Input: part model. Units: mm. Frame: model coordinates. Face numbers are marked on the shaded views. Coordinates: 2 decimals unless noted, no trailing zeros. Loops run counter-clockwise (first coordinate to the right, second up) from the corner with the lowest first, then second, coordinate; pieces in that order, holes last.
(1) Section B-B, the plane z = -1866.5. Return loops of the section in (x, y).
(2) Mould query, pull axis Z, two halves, no side actions, for the marked faces 1, 2 and 3. Classes: released by +Z, released by -Z, zero draft, split by the parting line, or undercut.
(3) Section C-C, the plane y = 150.5. Return loops of the section in (x, z), then the cut area to 3 significant figures.
(4) Contact query for flat-ended pins moving along their axis: P1, Ø6, axis at x = -238.5, z = -1429, coming from the +Y side; P2, Ø9, axis at x = 432.5, z = -2165, coming from the -Y side; P3, Ø1, axis at x = 249.5, z = -976, coming from the -Y side; P4, Ø20, axis at x = -436, y = -102.5, coming from the +Z side. Output: stop coordinate, or through.
(5) Section A-A, the plane y = -201.5. Give the number of separate pieces and of enclosed holes in the cut face, then the cut area to 3 significant figures.
(6) Section D-D, the plane x = -172. Return loops of the section in (y, z), then the cut area to 3 significant figures.
(7) Line query: L1, parallel to Z at x = 66, y = 171.5; L2, parallel to Y at x = 334.5, z = -1180; L3, parallel to Z at x = -41, y = -112.5. Output: solid intervals per line, ascending.
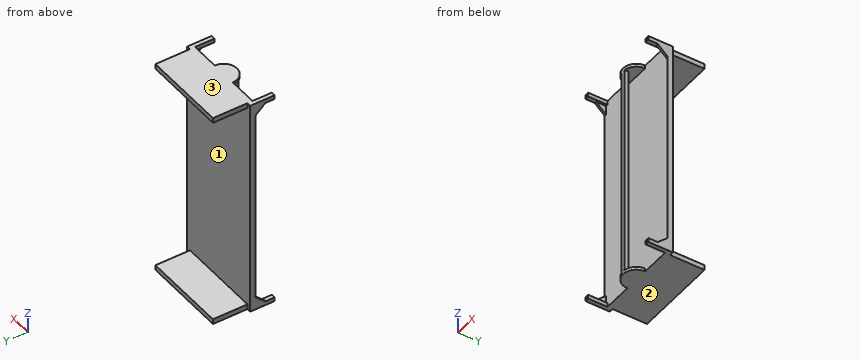
```python
from build123d import *

# Parameters (mm, degrees)
SKETCH1_W                = 40
SKETCH1_H                = 10
BOSS_EXTRUDE1_DEPTH      = 50
BOSS_EXTRUDE2_DEPTH      = 340
BOSS_EXTRUDE2_DEPTH_BACK = 50
SKETCH1_4_W              = 40
SKETCH1_4_H              = 40
BOSS_EXTRUDE3_DEPTH      = 240
BOSS_EXTRUDE4_DEPTH      = 20
BOSS_EXTRUDE5_DEPTH      = 20
SKETCH5_W                = 30
SKETCH5_H                = 30
CUT_EXTRUDE1_DEPTH       = 200
BOSS_EXTRUDE6_DEPTH      = 30
BOSS_EXTRUDE7_START      = -30
BOSS_EXTRUDE7_DEPTH      = 30
BOSS_EXTRUDE8_DEPTH      = 20
BOSS_EXTRUDE8_DEPTH_BACK = 20


with BuildPart() as part:
    # Sketch1 → Boss-Extrude1 (new body)
    with BuildSketch(Plane(origin=(0, 0, 0), x_dir=(1, 0, 0), z_dir=(0, 1, 0))):
        Polygon((-457.5, 50), (-417.5, 50), (417.5, 50), (457.5, 50), (457.5, 2130), (417.5, 2130), (-417.5, 2130), (-457.5, 2130), align=None)
        with Locations((-437.5, 45)):
            Rectangle(SKETCH1_W, SKETCH1_H)
        with Locations((437.5, 45)):
            Rectangle(SKETCH1_W, SKETCH1_H)
        with Locations((437.5, 2135)):
            Rectangle(SKETCH1_W, SKETCH1_H)
        with Locations((-437.5, 2135)):
            Rectangle(SKETCH1_W, SKETCH1_H)
    extrude(amount=-BOSS_EXTRUDE1_DEPTH)

    # Sketch1_3 → Boss-Extrude2 (add, two sides: drawn at the far end of the back side and taken through both)
    with BuildSketch(Plane(origin=(0, 0, 0), x_dir=(1, 0, 0), z_dir=(0, 1, 0)).offset(-BOSS_EXTRUDE2_DEPTH_BACK)):
        Polygon((-417.5, 50), (-417.5, 40), (-417.5, 0), (417.5, 0), (417.5, 40), (417.5, 50), align=None)
        Polygon((-417.5, 2140), (-417.5, 2130), (417.5, 2130), (417.5, 2140), (417.5, 2180), (-417.5, 2180), align=None)
    extrude(amount=BOSS_EXTRUDE2_DEPTH + BOSS_EXTRUDE2_DEPTH_BACK)

    # Sketch1_4 → Boss-Extrude3 (add)
    with BuildSketch(Plane(origin=(0, 0, 0), x_dir=(1, 0, 0), z_dir=(0, 1, 0))):
        with Locations((437.5, 2160)):
            Rectangle(SKETCH1_4_W, SKETCH1_4_H)
        with Locations((-437.5, 2160)):
            Rectangle(SKETCH1_4_W, SKETCH1_4_H)
        with Locations((-437.5, 20)):
            Rectangle(SKETCH1_4_W, SKETCH1_4_H)
        with Locations((437.5, 20)):
            Rectangle(SKETCH1_4_W, SKETCH1_4_H)
    extrude(amount=-BOSS_EXTRUDE3_DEPTH)

    # Sketch3 → Boss-Extrude4 (add)
    with BuildSketch(Plane(origin=(457.5, 0, 0), x_dir=(0, 0, -1), z_dir=(1, 0, 0))):
        Polygon((40, -50), (40, -150), (130, -50), align=None)
        Polygon((2140, -50), (2050, -50), (2140, -150), align=None)
    extrude(amount=-BOSS_EXTRUDE4_DEPTH)

    # Sketch4 → Boss-Extrude5 (add)
    with BuildSketch(Plane(origin=(-457.5, 0, -45.75), x_dir=(0, 0, -1), z_dir=(1, 0, 0))):
        Polygon((2094.25, -50), (2004.25, -50), (2094.25, -150), align=None)
        Polygon((-5.75, -50), (-5.75, -150), (84.25, -50), align=None)
    extrude(amount=BOSS_EXTRUDE5_DEPTH)

    # Sketch5 → Cut-Extrude1 (cut)
    with BuildSketch(Plane.XZ.offset(240)):
        with Locations((-437.5, -2160)):
            Rectangle(SKETCH5_W, SKETCH5_H)
        with Locations((437.5, -2160)):
            Rectangle(SKETCH5_W, SKETCH5_H)
        with Locations((437.5, -20)):
            Rectangle(SKETCH5_W, SKETCH5_H)
        with Locations((-437.5, -20)):
            Rectangle(SKETCH5_W, SKETCH5_H)
    extrude(amount=-CUT_EXTRUDE1_DEPTH, mode=Mode.SUBTRACT)

    # Sketch6 → Boss-Extrude6 (add)
    with BuildSketch(Plane.XY):
        with BuildLine():
            Line((130, -50), (-130, -50))
            ThreePointArc((-130, -50), (0, -180), (130, -50))
        make_face()
    extrude(amount=-BOSS_EXTRUDE6_DEPTH)

    # Sketch7 → Boss-Extrude7 (add)
    with BuildSketch(Plane(origin=(0, 0, -2180), x_dir=(-1, 0, 0), z_dir=(0, 0, -1)).offset(BOSS_EXTRUDE7_START)):
        with BuildLine():
            Line((130, -50), (-130, -50))
            ThreePointArc((-130, -50), (0, -180), (130, -50))
        make_face()
    extrude(amount=BOSS_EXTRUDE7_DEPTH)

    # 3DSketch1 → Boss-Extrude8 (add, two sides: drawn at the far end of the back side and taken through both)
    with BuildSketch(Plane(origin=(0, -180, -30), x_dir=(0, 0.018864566947613626, -0.9998220482235222), z_dir=(1, 0, 0)).offset(-BOSS_EXTRUDE8_DEPTH_BACK)):
        Polygon((0, 0), (0.754582678, 39.992881929), (2120.377324912, 0), (2119.622742234, -39.992881929), align=None)
    extrude(amount=BOSS_EXTRUDE8_DEPTH + BOSS_EXTRUDE8_DEPTH_BACK)


solid = part.part
```
Report:
1. outline: (-457.5, -50) - (457.5, -50) - (457.5, 0) - (-457.5, 0) - close; (-20, -180) - (20, -180) - (20, -140) - (-20, -140) - close
2. face 1: undercut
2. face 2: released by -Z
2. face 3: released by +Z
3. outline: (-417.5, -2180) - (417.5, -2180) - (417.5, -2130) - (-417.5, -2130) - close; (-417.5, -50) - (417.5, -50) - (417.5, 0) - (-417.5, 0) - close
3. area: 83,500 mm2
4. P1: stops at y = 0
4. P2: stops at y = -40
4. P3: stops at y = -50
4. P4: stops at z = 0
5. separate pieces: 4
5. enclosed holes: 4
5. area: 2,800 mm2
6. outline: (-50, -2180) - (340, -2180) - (340, -2130) - (0, -2130) - (0, -50) - (340, -50) - (340, 0) - (-50, 0) - close
6. area: 143,000 mm2
7. L1: z = -2180 to -2130, -50 to 0
7. L2: y = -50 to 0
7. L3: z = -2180 to -2150, -30 to 0
